```python
from build123d import *

# Parameters (mm, degrees)
BOSS_EXTRUDE1_DEPTH = 16
SKETCH2_R           = 4.575
CUT_EXTRUDE1_DEPTH  = 2
CUT_EXTRUDE2_DEPTH  = 18.867638344
CUT_EXTRUDE3_START  = -1.05
SKETCH4_W           = 9.1
SKETCH4_H           = 5
CUT_EXTRUDE3_DEPTH  = 1.05
SKETCH5_W           = 9.1
SKETCH5_H           = 2
CUT_EXTRUDE4_DEPTH  = 19.255204737


with BuildPart() as part:
    # Sketch1 → Boss-Extrude1 (new body)
    with BuildSketch(Plane.XY):
        Polygon((0, 0), (0, 0.95), (6, 0.95), (6, 0), (7.55, 0), (7.55, -0.8), (4.8, -3.55), (1.2, -3.55), (-1.55, -0.8), (-1.55, 0), align=None)
    extrude(amount=BOSS_EXTRUDE1_DEPTH)

    # Sketch2 → Cut-Extrude1 (cut)
    with BuildSketch(Plane(origin=(0, 0.95, 0), x_dir=(1, 0, 0), z_dir=(0, 1, 0))):
        with Locations((3, -8)):
            Circle(SKETCH2_R)
    extrude(amount=-CUT_EXTRUDE1_DEPTH, mode=Mode.SUBTRACT)

    # Sketch3 → Cut-Extrude2 (cut, through all)
    with BuildSketch(Plane(origin=(0, -1.05, 0), x_dir=(1, 0, 0), z_dir=(0, 1, 0))):
        Polygon((3, -4.766838493), (0.2, -6.383419246), (0.2, -9.616580754), (3, -11.233161507), (5.8, -9.616580754), (5.8, -6.383419246), align=None)
    extrude(amount=-CUT_EXTRUDE2_DEPTH, mode=Mode.SUBTRACT)

    # Sketch4 → Cut-Extrude3 (cut)
    with BuildSketch(Plane(origin=(0, 0, 0), x_dir=(1, 0, 0), z_dir=(0, 1, 0)).offset(CUT_EXTRUDE3_START)):
        with Locations((3, -8)):
            Rectangle(SKETCH4_W, SKETCH4_H)
    extrude(amount=CUT_EXTRUDE3_DEPTH, mode=Mode.SUBTRACT)

    # Sketch5 → Cut-Extrude4 (cut, through all)
    with BuildSketch(Plane(origin=(0, 0.95, 0), x_dir=(1, 0, 0), z_dir=(0, 1, 0))):
        with Locations((3, -1)):
            Rectangle(SKETCH5_W, SKETCH5_H)
        with Locations((3, -15)):
            Rectangle(SKETCH5_W, SKETCH5_H)
    extrude(amount=-CUT_EXTRUDE4_DEPTH, mode=Mode.SUBTRACT)


solid = part.part
```
Source: CAD feature listing. Evaluate the final solid. Frame: model axes, mm. A direction names the side the tool comes from. Give positions to 0.01 mm unless a question says otherwise; leave off trailing zeros. Loops run counter-clockwise (first coordinate to the right, second up) from the corner with the lowest first, then second, coordinate; pieces in that order, holes last. Notation, with made-up numbers: (-7, 48.5) -> (3, 48.5) arc R8 cw to (3, 54.5) -> close; hole circle Ø7 at (47.25, 17). An arc over 180 degrees is marked (long way). Put each result on its own line as item: value. Start each with the question number.
1) Contact query for flat-ended pins moving along their axis: P1, Ø1.2, axis at y = -2, z = 8.5, coming from the +X side; P2, Ø0.8, axis at x = 7, z = 12, coming from the +Y side; P3, Ø0.5, axis at y = 0.5, z = 3, coming from the +X side. Output: stop coordinate, or through.
2) Cut plane B-B (z = 8.5). Return loops of the section in (x, y), then the cut area to 3 significant figures.
3) Cut plane A-A (y = -0.3). Return loops of the section in (x, z) (3 decimals).
4) Cut plane D-D (x = 1.5). Return loops of the section in (y, z), then the cut area to 3 significant figures.
5) Material intervals for probe 1 along Y at (x, z) = (3.25, 11.5); probe 2 along Z at (x, y) = (4.5, -1); probe 3 along Z at (x, y) = (1, -2.05), sorted ascending.
6) Draft query along X for faces 1 (the face through (0.2, -2, 8)), 2 (the face through (3, -1, 2)), 3 (the face through (6.19, -2.16, 7.92)). Return one class per face: released by +X, released by -X, zero draft, split by the parting line, or undercut.
7) Reachability of faces 4 (the face through (5.8, -2, 8)), 5 (the face through (-1, 0, 4)), 6 (the face through (6, 0.5, 12.7)) from +Z, -Z, +X, -X, +Y, -Y: full face, straight path, thin tool, end or side. Return the list, or none.
8) Cut plane C-C (y = -2.1). Return loops of the section in (x, z).
Results are:
1. P1: stops at x = 6.95
1. P2: stops at y = 0
1. P3: stops at x = 6
2. outline: (-1.3, -1.05) -> (0.2, -2.55) -> (0.2, -1.05) -> close; (5.8, -2.55) -> (7.3, -1.05) -> (5.8, -1.05) -> close
2. area: 2.25 mm2
3. outline: (-1.55, 2) -> (7.55, 2) -> (7.55, 5.5) -> (6.832, 5.5) arc R4.575 cw to (-0.832, 5.5) -> (-1.55, 5.5) -> close; (-1.55, 10.5) -> (-0.832, 10.5) arc R4.575 cw to (6.832, 10.5) -> (7.55, 10.5) -> (7.55, 14) -> (-1.55, 14) -> close
4. outline: (-3.55, 2) -> (0.95, 2) -> (0.95, 3.68) -> (-1.05, 3.68) -> (-1.05, 5.63) -> (-3.55, 5.63) -> close; (-3.55, 10.37) -> (-1.05, 10.37) -> (-1.05, 12.32) -> (0.95, 12.32) -> (0.95, 14) -> (-3.55, 14) -> close
4. area: 24.9 mm2
5. probe 1: y = -3.55 to -1.05
5. probe 2: z = 2 to 3.68, 12.32 to 14
5. probe 3: z = 2 to 5.92, 10.08 to 14
6. face 1: undercut
6. face 2: zero draft
6. face 3: released by +X
7. face 4: +Y, -Y
7. face 5: +Z, -Z, -X, +Y
7. face 6: +Z, -Z, +X, +Y
8. outline: (-0.25, 2) -> (6.25, 2) -> (6.25, 14) -> (-0.25, 14) -> close; hole (0.2, 6.38) -> (3, 4.77) -> (5.8, 6.38) -> (5.8, 9.62) -> (3, 11.23) -> (0.2, 9.62) -> close
